```python
from build123d import *

# Parameters (mm, degrees)
PAD_DEPTH   = 15
SKETCH001_R = 2
HOLE_DEPTH  = 25


with BuildPart() as part:
    # Sketch → Pad (new body)
    with BuildSketch(Plane.XY):
        Polygon((-4.425698, 71.54545), (-4.425698, 51.54545), (-37.425698, 51.54545), (-37.425698, -11.45455), (-4.425698, -11.45455), (-4.425698, -31.45455), (0.574302, -31.45455), (0.574302, -8.45455), (-34.425698, -8.45455), (-34.425698, 48.54545), (0.574302, 48.54545), (0.574302, 71.54545), align=None)
    extrude(amount=PAD_DEPTH)

    # Sketch001 (on Face5 of Pad) → Hole (cut)
    with BuildSketch(Plane(origin=(-4.425698, 0, 0), x_dir=(0, -1, 0), z_dir=(-1, 0, 0))):
        with Locations((-62.718771, 7)):
            Circle(SKETCH001_R)
        with Locations((23.384939, 7)):
            Circle(SKETCH001_R)
    extrude(amount=-HOLE_DEPTH, mode=Mode.SUBTRACT)


solid = part.part
```
Input: part model. Units: mm. Frame: model coordinates. A direction names the side the tool comes from. Give positions to 0.01 mm unless a question says otherwise; leave off trailing zeros. Write each loop counter-clockwise with the first axis right and the second up, starting at its lowest first coordinate (ties: lowest second). Pieces come first, ordered by that corner, then holes. Notation, with made-up numbers: (63.5, -31.75) - (95.5, -31.75) arc R20 cw to (95.5, -22.75) - close; hole circle Ø2 at (24, 64.5). An arc over 180 degrees is marked (long way). Write item = value, one per line. Start each with the question number.
1. Mould query, pull axis Y, two halves, no side actions, for faces 1 (the flat face through (-2, 71.545, 7)), 2 (the flat face through (-4.426, -21, 7)), 3 (the cylindrical face through (-1.961, -25.293, 7.601)). Classes: released by +Y, released by -Y, zero draft, split by the parting line, or undercut.
2. First-contact query: pin 1 Ø6 at (x, z) = (-9.5, 2) entering from -Y; pin 2 Ø1 at (x, z) = (-20.5, 1.5) entering from +Y; pin 3 Ø4.5 at (y, z) = (16, 9) entering from +X. Flat tips, straight axial feed; report the tip coordinate or a pass-through.
3. Section query C-C, the plane y = -23. Output: boundary loops of the cut face in (x, z).
4. Section query B-B, the plane x = -9.5. Output: boundary loops of the cut face in (y, z), then the cut area to 3 significant figures.
5. Access query for faces 4 (the flat face through (-17, -8.455, 7)), 5 (the flat face through (-4.426, 61.7, 9.1)), 6 (the flat face through (-21, -11.455, 7)). Directions: +Z, -Z, +X, -X, +Y, -Y. A direction counts if a zero-diameter tool reaches every point of the face in a straight line with its end or side. Return the directions, or none.
6. Section query A-A, the plane z = 7. Output: boundary loops of the cut face in (x, y), then the cut area to 3 significant figures.
7. Section query D-D, the plane z = 13. Output: boundary loops of the cut face in (x, y), then the cut area to 3 significant figures.
8. Ray query, L1, parallel to Y at x = -33, z = 6.75; L2, parallel to X at y = -2.5, z = 8; L3, parallel to X at y = -15.5, z = 14. Return the intervals inside material, ascending.
Check sheet entries:
q1.face_1 = released by +Y
q1.face_2 = zero draft
q1.face_3 = undercut
q2.pin_1 = -11.45
q2.pin_2 = 51.55
q2.pin_3 = -34.43
q3.outline = (-4.43, 0) - (0.57, 0) - (0.57, 5.04) - (-4.43, 5.04) - close; (-4.43, 8.96) - (0.57, 8.96) - (0.57, 15) - (-4.43, 15) - close
q4.outline = (-11.45, 0) - (-8.45, 0) - (-8.45, 15) - (-11.45, 15) - close; (48.55, 0) - (51.55, 0) - (51.55, 15) - (48.55, 15) - close
q4.area = 90.0 mm2
q5.face_4 = +Z, -Z, +X
q5.face_5 = +Z, -Z, -X, +Y
q5.face_6 = +Z, -Z, -X, -Y
q6.outline = (-37.43, -11.45) - (-4.43, -11.45) - (-4.43, -21.38) - (0.57, -21.38) - (0.57, -8.45) - (-34.43, -8.45) - (-34.43, 48.55) - (0.57, 48.55) - (0.57, 60.72) - (-4.43, 60.72) - (-4.43, 51.55) - (-37.43, 51.55) - close; (-4.43, -31.45) - (0.57, -31.45) - (0.57, -25.38) - (-4.43, -25.38) - close; (-4.43, 64.72) - (0.57, 64.72) - (0.57, 71.55) - (-4.43, 71.55) - close
q6.area = 559 mm2
q7.outline = (-37.43, -11.45) - (-4.43, -11.45) - (-4.43, -31.45) - (0.57, -31.45) - (0.57, -8.45) - (-34.43, -8.45) - (-34.43, 48.55) - (0.57, 48.55) - (0.57, 71.55) - (-4.43, 71.55) - (-4.43, 51.55) - (-37.43, 51.55) - close
q7.area = 599 mm2
q8.L1 = -11.45 to -8.45, 48.55 to 51.55
q8.L2 = -37.43 to -34.43
q8.L3 = -4.43 to 0.57
